```python
from build123d import *

# Parameters (mm, degrees)
SKETCH1_R           = 1.89865
SKETCH1_R_2         = 1.4732
BOSS_EXTRUDE3_DEPTH = 6.0452
SKETCH7_R           = 1.4732
CUT_EXTRUDE2_DEPTH  = 99.546673139
SKETCH9_R           = 1.4732
SKETCH9_W           = 30.226
SKETCH9_H           = 47.117
CUT_EXTRUDE3_DEPTH  = 14.732
SKETCH10_R          = 2.54
SKETCH10_W          = 5.7404
SKETCH10_H          = 2.8194
SKETCH10_W_2        = 2.8194
SKETCH10_H_2        = 5.7404
CUT_EXTRUDE4_DEPTH  = 6.0452


with BuildPart() as part:
    # Sketch1 → Boss-Extrude3 (new body)
    with BuildSketch(Plane.XY):
        with BuildLine():
            Line((-63.638843042, 39.6875), (-55.88, 39.6875))
            Line((-55.88, 39.6875), (-55.88, -39.6875))
            Line((-55.88, -39.6875), (-63.638843042, -39.6875))
            ThreePointArc((-63.638843042, -39.6875), (0, -75), (63.638843042, -39.6875))
            Line((63.638843042, -39.6875), (55.88, -39.6875))
            Line((55.88, -39.6875), (55.88, 39.6875))
            Line((55.88, 39.6875), (63.638843042, 39.6875))
            ThreePointArc((63.638843042, 39.6875), (50.33136084, 55.603544096), (33.172661219, 67.264957799))
            ThreePointArc((33.172661219, 67.264957799), (0, 47.904876359), (-33.172661219, 67.264957799))
            ThreePointArc((-33.172661219, 67.264957799), (-50.33136084, 55.603544096), (-63.638843042, 39.6875))
        make_face()
        with Locations((0, -66.675)):
            Circle(SKETCH1_R, mode=Mode.SUBTRACT)
        with Locations((-44.45, 49.6966108)):
            Circle(SKETCH1_R, mode=Mode.SUBTRACT)
        with Locations(Location((44.45, 49.6966108, 0), (0, 0, 180))):
            Circle(SKETCH1_R, mode=Mode.SUBTRACT)
        with Locations((-24.13, -15.875)):
            Circle(SKETCH1_R_2, mode=Mode.SUBTRACT)
        with Locations((-8.89, -15.875)):
            Circle(SKETCH1_R_2, mode=Mode.SUBTRACT)
        with Locations(Location((8.89, -15.875, 0), (0, 0, 180))):
            Circle(SKETCH1_R_2, mode=Mode.SUBTRACT)
        with Locations((-15.24, -65.475)):
            Circle(SKETCH1_R_2, mode=Mode.SUBTRACT)
        with Locations(Location((15.24, -65.475, 0), (0, 0, 180))):
            Circle(SKETCH1_R_2, mode=Mode.SUBTRACT)
        with Locations(Location((24.13, -15.875, 0), (0, 0, 180))):
            Circle(SKETCH1_R_2, mode=Mode.SUBTRACT)
        with Locations((8.89, 15.875)):
            Circle(SKETCH1_R_2, mode=Mode.SUBTRACT)
        with Locations(Location((-8.89, 15.875, 0), (0, 0, 180))):
            Circle(SKETCH1_R_2, mode=Mode.SUBTRACT)
        with Locations((24.13, 15.875)):
            Circle(SKETCH1_R_2, mode=Mode.SUBTRACT)
        with Locations(Location((-24.13, 15.875, 0), (0, 0, 180))):
            Circle(SKETCH1_R_2, mode=Mode.SUBTRACT)
    extrude(amount=BOSS_EXTRUDE3_DEPTH)

    # Sketch7 → Cut-Extrude2 (cut, through all)
    with BuildSketch(Plane.XY.offset(6.0452)):
        with Locations(Location((-31.75, -41.98, 0), (0, 0, 180))):
            Circle(SKETCH7_R)
        with Locations((31.75, -41.98)):
            Circle(SKETCH7_R)
    extrude(amount=-CUT_EXTRUDE2_DEPTH, mode=Mode.SUBTRACT)

    # Sketch9 → Cut-Extrude3 (cut)
    with BuildSketch(Plane.XY.offset(6.0452)):
        with Locations((-16.51, 45.301376359)):
            Circle(SKETCH9_R)
        with Locations((16.51, 45.301376359)):
            Circle(SKETCH9_R)
        with Locations((-16.51, -9.308623641)):
            Circle(SKETCH9_R)
        with Locations((16.51, -9.308623641)):
            Circle(SKETCH9_R)
        with Locations((0, 17.996376359)):
            Rectangle(SKETCH9_W, SKETCH9_H)
    extrude(amount=-CUT_EXTRUDE3_DEPTH, mode=Mode.SUBTRACT)

    # Sketch10 → Cut-Extrude4 (cut)
    with BuildSketch(Plane.XY.offset(6.0452)):
        with Locations((-38.735, -52.3875)):
            Circle(SKETCH10_R)
        with Locations((38.735, -52.3875)):
            Circle(SKETCH10_R)
        with Locations((-38.1, 51.1175)):
            Circle(SKETCH10_R)
        with Locations((38.1, 51.1175)):
            Circle(SKETCH10_R)
        with Locations((-38.1, 58.7375)):
            Rectangle(SKETCH10_W, SKETCH10_H)
        with Locations((38.1, 58.7375)):
            Rectangle(SKETCH10_W, SKETCH10_H)
        with Locations((-46.355, -52.3875)):
            Rectangle(SKETCH10_W_2, SKETCH10_H_2)
        with Locations((46.355, -52.3875)):
            Rectangle(SKETCH10_W_2, SKETCH10_H_2)
    extrude(amount=-CUT_EXTRUDE4_DEPTH, mode=Mode.SUBTRACT)


solid = part.part
```
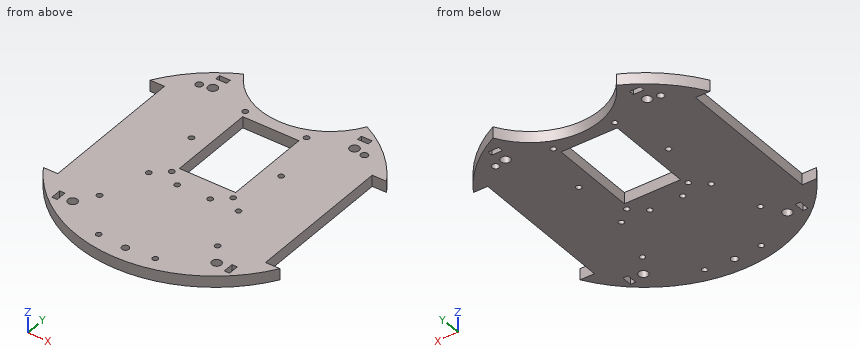
Read the model definition and answer for the solid it produces. Units are mm, in the model's axes. Give positions to 0.01 mm unless a question says otherwise; leave off trailing zeros. Write each loop counter-clockwise with the first axis right and the second up, starting at its lowest first coordinate (ties: lowest second). Pieces come first, ordered by that corner, then holes. Notation, with made-up numbers: (24, 81.25) -> (81, 81.25) arc R16 ccw to (81, 100.25) -> close; hole circle Ø6 at (46.5, 36). An arc over 180 degrees is marked (long way). Answer in a Markdown table with one row per item.
1) Each of these flat-tipped pins is pushed along its axis until it touches: pin 1 Ø3 at (y, z) = (-6.5, 2) entering from -X; pin 2 Ø3 at (x, z) = (-3, 1.5) entering from +Y; pin 3 Ø1 at (y, z) = (-48, 5.5) entering from -X. Where does it stop, or does it pass through?
Results list:
| item | result |
|---|---|
| pin 1 | x = -55.88 |
| pin 2 | y = 48.17 |
| pin 3 | x = -58.04 |
2) Section A-A on y = 5.5 is taken. Give the vertices of the cut face in (x, z), plus the area to 3 significant figures.
Results list:
| item | result |
|---|---|
| outline | (-55.88, 0) -> (-15.11, 0) -> (-15.11, 6.05) -> (-55.88, 6.05) -> close; (15.11, 0) -> (55.88, 0) -> (55.88, 6.05) -> (15.11, 6.05) -> close |
| area | 493 mm^2 |
3) Section D-D on y = -20.5 is taken. Give the vertices of the cut face in (x, z), plus the area to 3 significant figures.
Results list:
| item | result |
|---|---|
| outline | (-55.88, 0) -> (55.88, 0) -> (55.88, 6.05) -> (-55.88, 6.05) -> close |
| area | 676 mm^2 |
4) Straight lines are drawn through the part: line 1 (X direction, y = -5.5, z = 4); line 2 (X direction, y = -66.5, z = 5.25); line 3 (X direction, y = -54.5, z = 0.5). For each, find the intervals that lie inside material, in ascending order. Write a range as [from, to].
Results list:
| item | result |
|---|---|
| line 1 | [-55.88, -15.11], [15.11, 55.88] |
| line 2 | [-34.68, -16.3], [-14.18, -1.89], [1.89, 14.18], [16.3, 34.68] |
| line 3 | [-51.52, -47.76], [-44.95, -40.15], [-37.32, 37.32], [40.15, 44.95], [47.76, 51.52] |
5) Section B-B on x = 0 is taken. Give the vertices of the cut face in (y, z).
Results list:
| item | result |
|---|---|
| outline | (-75, 0) -> (-68.57, 0) -> (-68.57, 6.05) -> (-75, 6.05) -> close; (-64.78, 0) -> (-5.56, 0) -> (-5.56, 6.05) -> (-64.78, 6.05) -> close; (41.55, 0) -> (47.9, 0) -> (47.9, 6.05) -> (41.55, 6.05) -> close |
6) Section C-C on x = -38.1 is taken. Give the vertices of the cut face in (y, z).
Results list:
| item | result |
|---|---|
| outline | (-64.6, 0) -> (-54.85, 0) -> (-54.85, 6.05) -> (-64.6, 6.05) -> close; (-49.93, 0) -> (48.58, 0) -> (48.58, 6.05) -> (-49.93, 6.05) -> close; (53.66, 0) -> (57.33, 0) -> (57.33, 6.05) -> (53.66, 6.05) -> close; (60.15, 0) -> (64.6, 0) -> (64.6, 6.05) -> (60.15, 6.05) -> close |
